Geometry check sheet. Reference: drawing and pictorial views, mm from the part's lowest x, y, z. Give positions to 0.01 mm unless a question says otherwise; leave off trailing zeros. Write each loop counter-clockwise with the first axis right and the second up, starting at its lowest first coordinate (ties: lowest second). Pieces come first, ordered by that corner, then holes. Notation, with made-up numbers: (56, 32.5) -> (66, 32.5) arc R19 cw to (66, 47.5) -> close; hole circle Ø10 at (65.5, 73). An arc over 180 degrees is marked (long way). Return JSON: item names as keys, results as strings.
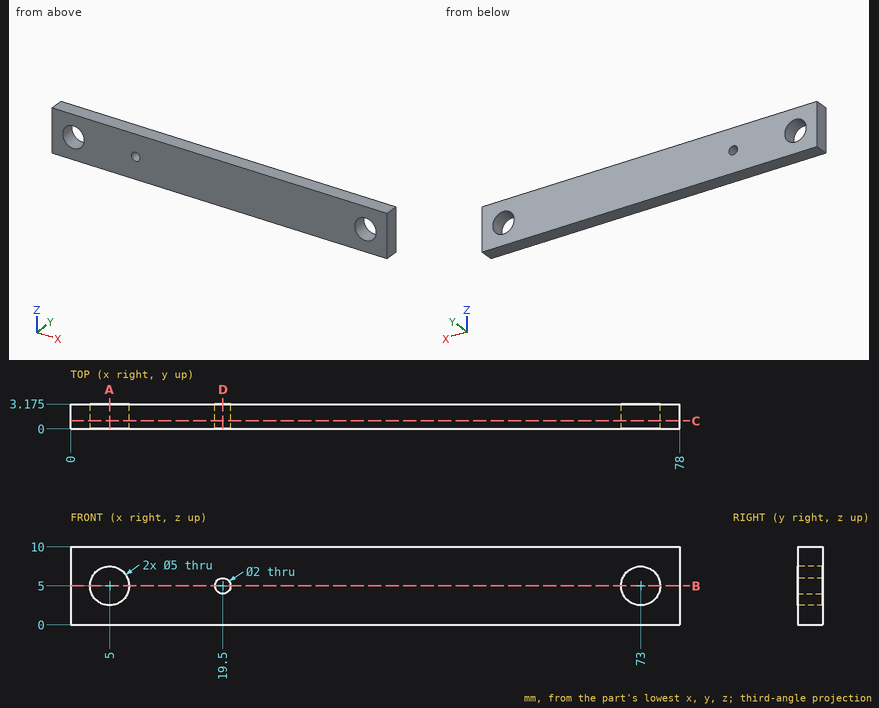
(1) Thickness scan on L1, parallel to X at y = 2.3, z = 5; L2, parallel to X at y = 1.3, z = 2.75; L3, parallel to Z at x = 73, y = 1.5. Record the ranges inside material, lowest first.
Reply:
{"L1": "0 to 2.5, 7.5 to 18.5, 20.5 to 70.5, 75.5 to 78", "L2": "0 to 3.91, 6.09 to 71.91, 74.09 to 78", "L3": "0 to 2.5, 7.5 to 10"}
(2) Cross-section at D-D on x = 19.5. Enter the section's corners in (y, z) (3 decimals).
Reply:
{"outline": "(0, 0) -> (3.175, 0) -> (3.175, 4) -> (0, 4) -> close; (0, 6) -> (3.175, 6) -> (3.175, 10) -> (0, 10) -> close"}
(3) Cross-section at C-C on y = 1. Enter the section's corners in (x, z).
Reply:
{"outline": "(0, 0) -> (78, 0) -> (78, 10) -> (0, 10) -> close; hole circle Ø5 at (5, 5); hole circle Ø2 at (19.5, 5); hole circle Ø5 at (73, 5)"}
(4) Cross-section at B-B on z = 5. Enter the section's corners in (x, y) (3 decimals).
Reply:
{"outline": "(0, 0) -> (2.5, 0) -> (2.5, 3.175) -> (0, 3.175) -> close; (7.5, 0) -> (18.5, 0) -> (18.5, 3.175) -> (7.5, 3.175) -> close; (20.5, 0) -> (70.5, 0) -> (70.5, 3.175) -> (20.5, 3.175) -> close; (75.5, 0) -> (78, 0) -> (78, 3.175) -> (75.5, 3.175) -> close"}
(5) Cross-section at A-A on x = 5. Enter the section's corners in (y, z) (3 decimals), then the cut area to 3 significant figures.
Reply:
{"outline": "(0, 0) -> (3.175, 0) -> (3.175, 2.5) -> (0, 2.5) -> close; (0, 7.5) -> (3.175, 7.5) -> (3.175, 10) -> (0, 10) -> close", "area": "15.9 mm^2"}
